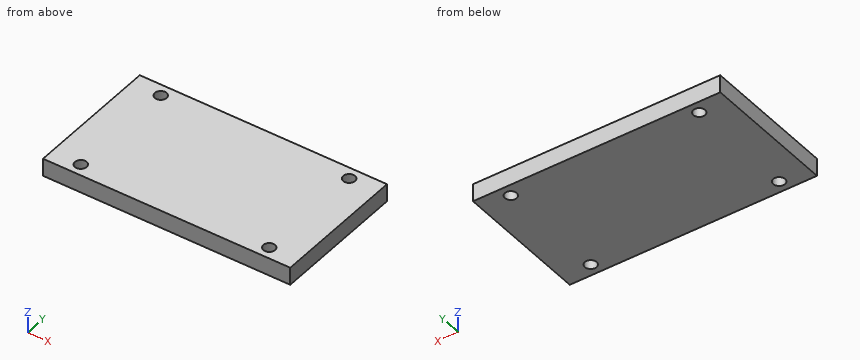
Autodesk Inventor part; units mm, degrees
ref_plane "YZ Plane" through (0, 0, 0) normal (1, 0, 0) x (0, 1, 0)
ref_plane "XZ Plane" through (0, 0, 0) normal (0, 1, 0) x (-1, 0, 0)
ref_plane "XY Plane" through (0, 0, 0) normal (0, 0, 1) x (1, 0, 0)
sketch "Эскиз1" plane through (0, 0, 0) normal (0, 0, 1) x (1, 0, 0)
  line L0 (-21, -11.5) -> (21, -11.5)
  line L1 (21, -11.5) -> (21, 11.5)
  line L2 (21, 11.5) -> (-21, 11.5)
  line L3 (-21, 11.5) -> (-21, -11.5)
  line L4 (-21, -11.5) -> (21, 11.5) construction
  line L5 (21, -11.5) -> (-21, 11.5) construction
  line L6 (21, -11.5) -> (16, -11.5) construction
  line L7 (16, -11.5) -> (16, -9.5) construction
  line L8 (-21, 11.5) -> (-16, 11.5) construction
  line L9 (-16, 11.5) -> (-16, 9.5) construction
  circle A0 centre (-16, 9.5) radius 1
  circle A1 centre (16, -9.5) radius 1
  line L10 (0, 11.5) -> (0, -11.5) construction
  circle A2 centre (16, 9.5) radius 1
  circle A3 centre (-16, -9.5) radius 1
  point P0 (0, 0)
  dimension "d0" = 42
  dimension "d1" = 23
  dimension "d2" = 5
  dimension "d3" = 2
  dimension "d4" = 5
  dimension "d5" = 2
  dimension "d6" = 2
  dimension "d7" = 2
extrude "Выдавливание1" add sketch "Эскиз1" along normal blind 3
Input: part model. Units: mm. Frame: model coordinates. Round coordinates to 2 decimals unless told otherwise and drop trailing zeros. Loops run counter-clockwise (first coordinate to the right, second up) from the corner with the lowest first, then second, coordinate; pieces in that order, holes last. Notation, with made-up numbers: (74.5, 65.25) - (113.5, 65.25) arc R11 ccw to (113.5, 76.25) - close; hole circle Ø8 at (89.5, -23.75). An arc over 180 degrees is marked (long way). One line per item, written item: value. Start each with the question number.
(1) Ray query, line 1 (Y direction, x = 16, z = 2.05); line 2 (X direction, y = 10.25, z = 2.1). Return the intervals inside material, ascending. Write a range as [from, to].
(2) Contact query for flat-ended pins moving along their axis: P1, Ø1.8, axis at x = -16, y = -9.5, coming from the +Z side; P2, Ø2.5, axis at x = 16, y = -9.5, coming from the -Z side. Output: stop coordinate, or through.
(3) Section B-B, the plane x = -16. Return loops of the section in (y, z).
(4) Section A-A, the plane y = 9.5. Return loops of the section in (x, z).
Results below:
1. line 1: [-11.5, -10.5], [-8.5, 8.5], [10.5, 11.5]
1. line 2: [-21, -16.66], [-15.34, 15.34], [16.66, 21]
2. P1: through
2. P2: z = 0
3. outline: (-11.5, 0) - (-10.5, 0) - (-10.5, 3) - (-11.5, 3) - close; (-8.5, 0) - (8.5, 0) - (8.5, 3) - (-8.5, 3) - close; (10.5, 0) - (11.5, 0) - (11.5, 3) - (10.5, 3) - close
4. outline: (-21, 0) - (-17, 0) - (-17, 3) - (-21, 3) - close; (-15, 0) - (15, 0) - (15, 3) - (-15, 3) - close; (17, 0) - (21, 0) - (21, 3) - (17, 3) - close
